Can you work these out from the model? Positions are in its coordinate system, mm. A direction names the side the tool comes from. Give positions to 0.01 mm unless a question says otherwise; leave off trailing zeros. Loops run counter-clockwise (first coordinate to the right, second up) from the corner with the lowest first, then second, coordinate; pieces in that order, holes last. Notation, with made-up numbers: (27.5, 54) - (80.5, 54) arc R9 cw to (80.5, 64) - close; hole circle Ø11 at (61, 78). An arc over 180 degrees is marked (long way). Answer as a JSON object with one key per item and string values. Group by question number.
Item 1: Please list where these lines run through material, in increasing order: L1, parallel to X at y = -14.5, z = 8.5; L2, parallel to X at y = -12.5, z = 7.4; L3, parallel to Y at x = 3, z = 4.
Item 2: Which directions (+Z, -Z, +X, -X, +Y, -Y) give clear straight access to the entire face, cutting with the end or side of a thin tool? Please do faces 1 (the flat face through (-37.78, -6.91, 5.18)), 2 (the cylindrical face through (2.66, -35.22, 5.18)), 3 (the cylindrical face through (2.5, 37.4, 5.2)), 4 (the cylindrical face through (7.85, -3.45, 8.04)).
Item 3: Suppose I cut it at D-D on y = -5. Write out the boundary of the cut face in (x, z), and give its area (3 significant figures).
Item 4: Thinking about a two-plate mould opening in Y: for faces 5 (the flat face through (9, -5, 5.5)), 6 (the flat face through (0, 10, 5.5)), 7 (the flat face through (-24.987, -29.067, 5.176)), which applies, pulls with the +Y half, pulls with the -Y half, needs draft (parallel to the pull), parting line crosses it, or undercut?
Item 5: Will these pins go through, and if not, where does the flat tip stop? pin 1 (2 mm diameter, centred on y = -0.5, z = 4.5, fed in from -X); pin 2 (1 mm diameter, centred on x = -9, y = -4.5, fed in from +Z); pin 3 (6 mm diameter, centred on y = 15.5, z = 5, fed in from -X); pin 4 (11 mm diameter, centred on x = 1.5, y = 27.5, fed in from +Z).
Item 6: Suppose I cut it at C-C on y = 10. Write out the boundary of the cut face in (x, z), and give its area (3 significant figures).
Item 7: Suppose I cut it at A-A on x = 0. Write out the boundary of the cut face in (y, z), and give its area (3 significant figures).
Autodesk Fusion 360 part; units mm, degrees
sketch "Sketch1" plane through (0, 0, 0) normal (0, 0, 1) x (1, 0, 0)
  line L0 (42, 0) -> (21, 36.3731)
  line L1 (21, 36.3731) -> (-21, 36.3731)
  line L2 (-21, 36.3731) -> (-42, 0)
  line L3 (-42, 0) -> (-21, -36.3731)
  line L4 (-21, -36.3731) -> (21, -36.3731)
  line L5 (21, -36.3731) -> (42, 0)
  circle A0 centre (0, 42.3731) radius 4
  line L6 (0, 41) -> (0, 36.3731)
  arc A1 (2.9814, 39.7064) -> (4.4721, 36.3731) centre (4.4721, 38.3731) ccw
  arc A2 (-4.4721, 36.3731) -> (-2.9814, 39.7064) centre (-4.4721, 38.3731) ccw
  circle A3 centre (-36.6962, -21.1865) radius 4
  arc A4 (-29.2639, -22.0595) -> (-32.896, -22.4352) centre (-30.996, -23.0595) ccw
  arc A5 (-35.8775, -17.2712) -> (-33.7361, -14.3136) centre (-35.4681, -15.3136) ccw
  circle A6 centre (36.6962, -21.1865) radius 4
  arc A7 (33.7361, -14.3136) -> (35.8775, -17.2712) centre (35.4681, -15.3136) ccw
  arc A8 (32.896, -22.4352) -> (29.2639, -22.0595) centre (30.996, -23.0595) ccw
  circle A9 centre (-26.3038, 15.1865) radius 4
  arc A10 (-29.2639, 22.0595) -> (-27.1225, 19.1019) centre (-27.5319, 21.0595) ccw
  arc A11 (-30.104, 13.9379) -> (-33.7361, 14.3136) centre (-32.004, 13.3136) ccw
  circle A12 centre (0, -30.3731) radius 4
  arc A13 (-4.4721, -36.3731) -> (-2.9814, -33.0397) centre (-4.4721, -34.3731) ccw
  arc A14 (2.9814, -33.0397) -> (4.4721, -36.3731) centre (4.4721, -34.3731) ccw
  circle A15 centre (26.3038, 15.1865) radius 4
  arc A16 (33.7361, 14.3136) -> (30.104, 13.9379) centre (32.004, 13.3136) ccw
  arc A17 (27.1225, 19.1019) -> (29.2639, 22.0595) centre (27.5319, 21.0595) ccw
  dimension "d1" = 42
  dimension "d2" = 8
  dimension "d3" = 6
  dimension "d4" = 4
  dimension "d6" = 360
  dimension "d10" = 360
extrude "Extrude1" add sketch "Sketch1" along normal blind 10.5 contours L0 L1 L2 L3 L4 L5 A9 A10 A11 A12 A13 A14 A15 A16 A17 | L5 A6 A7 A8 | A6 | L1 A0 L6 A1 | L1 A0 L6 A2 | A0 | L3 A3 A4 A5 | A3
move_face "OffsetFaces1" offset -0.2 9 faces at (35.4632, -24.9918, 7) (29.3138, -21.9777, 7) (-37.9917, -24.9709, 7) (-30.5353, -21.1133, 7) (34.8369, -17.2113, 7) (-3.1097, 39.8571, 7) (2.513, 38.7754, 7) (-34.8369, -17.2113, 7) (-2.513, 38.7754, 7)
sketch "Sketch2" plane through (0, 0, 10.5) normal (0, 0, 1) x (-1, 0, 0)
  line L0 (-33.5629, 14.2136) -> (-41.8845, -0.2)
  line L1 (-41.8845, -0.2) -> (-33.7361, -14.3136)
  arc A0 (-33.7361, -14.3136) -> (-30.104, -13.9379) centre (-32.004, -13.3136) ccw
  arc A1 (-27.1225, -19.1019) -> (-30.104, -13.9379) centre (-26.3038, -15.1865) ccw
  arc A2 (-27.1225, -19.1019) -> (-29.2639, -22.0595) centre (-27.5319, -21.0595) ccw
  line L2 (-29.2639, -22.0595) -> (-21.1155, -36.1731)
  line L3 (-21.1155, -36.1731) -> (-4.4721, -36.1731)
  arc A3 (-2.8324, -39.8397) -> (-4.4721, -36.1731) centre (-4.4721, -38.3731) ccw
  arc A4 (-2.8324, -39.8397) -> (2.8324, -39.8397) centre (0, -42.3731) ccw
  arc A5 (4.4721, -36.1731) -> (2.8324, -39.8397) centre (4.4721, -38.3731) ccw
  line L4 (4.4721, -36.1731) -> (21.1155, -36.1731)
  line L5 (21.1155, -36.1731) -> (29.2639, -22.0595)
  arc A6 (29.2639, -22.0595) -> (27.1225, -19.1019) centre (27.5319, -21.0595) ccw
  arc A7 (30.104, -13.9379) -> (27.1225, -19.1019) centre (26.3038, -15.1865) ccw
  arc A8 (30.104, -13.9379) -> (33.7361, -14.3136) centre (32.004, -13.3136) ccw
  line L6 (33.7361, -14.3136) -> (41.8845, -0.2)
  line L7 (41.8845, -0.2) -> (33.5629, 14.2136)
  arc A9 (35.9184, 17.467) -> (33.5629, 14.2136) centre (35.4681, 15.3136) ccw
  arc A10 (35.9184, 17.467) -> (33.086, 22.3728) centre (36.6962, 21.1865) ccw
  arc A11 (29.0907, 21.9595) -> (33.086, 22.3728) centre (30.996, 23.0595) ccw
  line L8 (29.0907, 21.9595) -> (20.7691, 36.3731)
  line L9 (20.7691, 36.3731) -> (4.4721, 36.3731)
  arc A12 (4.4721, 36.3731) -> (2.9814, 33.0397) centre (4.4721, 34.3731) ccw
  arc A13 (-2.9814, 33.0397) -> (2.9814, 33.0397) centre (0, 30.3731) ccw
  arc A14 (-2.9814, 33.0397) -> (-4.4721, 36.3731) centre (-4.4721, 34.3731) ccw
  line L10 (-4.4721, 36.3731) -> (-20.7691, 36.3731)
  line L11 (-20.7691, 36.3731) -> (-29.0907, 21.9595)
  arc A15 (-33.086, 22.3728) -> (-29.0907, 21.9595) centre (-30.996, 23.0595) ccw
  arc A16 (-33.086, 22.3728) -> (-35.9184, 17.467) centre (-36.6962, 21.1865) ccw
  arc A17 (-33.5629, 14.2136) -> (-35.9184, 17.467) centre (-35.4681, 15.3136) ccw
  circle A18 centre (0, -25) radius 10
  circle A19 centre (0, -25) radius 5
  circle A20 centre (0, -10) radius 1.75
  circle A21 centre (21.6506, 12.5) radius 5
  circle A22 centre (21.6506, 12.5) radius 10
  circle A23 centre (-21.6506, 12.5) radius 5
  circle A24 centre (-21.6506, 12.5) radius 10
  circle A25 centre (8.6603, -5) radius 1.75
  circle A26 centre (8.6603, 5) radius 1.75
  circle A27 centre (0, 10) radius 1.75
  circle A28 centre (-8.6603, 5) radius 1.75
  circle A29 centre (-8.6603, -5) radius 1.75
  dimension "d14" = 10
  dimension "d15" = 20
  dimension "d16" = 3.5
  dimension "d18" = 360
  dimension "d20" = 360
extrude "Extrude2" cut sketch "Sketch2" against normal blind 1.5 contours A18 | A22 | A24
extrude "Extrude3" cut 3 faces at (-2.3344, 25.4913, 10.5) (-21.8157, -11.3785, 10.5) (21.4856, -11.3785, 10.5) along direction (0, 0, -1) blind 6
extrude "Extrude4" cut sketch "Sketch2" against normal blind 5 contours A20 | A25 | A26 | A27 | A28 | A29
Worked out:
{
 "1": {"L1": "x = -33.42 to -26.23, -17.07 to 17.07, 26.23 to 33.42", "L2": "x = -34.55 to -26.65, -16.65 to 16.65, 26.65 to 34.55", "L3": "y = -35.73 to -33.02, -27.73 to 36.74, 40.04 to 44.71"},
 "2": {"face 1": "+Z, -Z, -X", "face 2": "+Z, -Z", "face 3": "+Z, -Z, +X", "face 4": "+Z"},
 "3": {"outline": "(-38.88, 0) - (38.88, 0) - (38.88, 10.5) - (28.26, 10.5) - (28.26, 9) - (15.04, 9) - (15.04, 10.5) - (10.41, 10.5) - (10.41, 5.5) - (6.91, 5.5) - (6.91, 10.5) - (-6.91, 10.5) - (-6.91, 5.5) - (-10.41, 5.5) - (-10.41, 10.5) - (-15.04, 10.5) - (-15.04, 9) - (-28.26, 9) - (-28.26, 10.5) - (-38.88, 10.5) - close", "area": "742 mm2"},
 "4": {"face 5": "undercut", "face 6": "undercut", "face 7": "pulls with the -Y half"},
 "5": {"pin 1": "stops at x = -41.88", "pin 2": "stops at z = 5.5", "pin 3": "stops at x = -34.78", "pin 4": "stops at z = 9"},
 "6": {"outline": "(-36.23, 0) - (36.23, 0) - (36.23, 10.5) - (1.75, 10.5) - (1.75, 5.5) - (-1.75, 5.5) - (-1.75, 10.5) - (-36.23, 10.5) - close", "area": "743 mm2"},
 "7": {"outline": "(-26.37, 0) - (46.17, 0) - (46.17, 10.5) - (35, 10.5) - (35, 9) - (30, 9) - (30, 4.5) - (20, 4.5) - (20, 9) - (15, 9) - (15, 10.5) - (11.75, 10.5) - (11.75, 5.5) - (8.25, 5.5) - (8.25, 10.5) - (-8.25, 10.5) - (-8.25, 5.5) - (-11.75, 5.5) - (-11.75, 10.5) - (-26.37, 10.5) - close", "area": "652 mm2"}
}
